Build history of the part. All positions in model axes, mm. A direction names the side the tool comes from. Coordinates: 2 decimals unless noted, no trailing zeros. Write each loop counter-clockwise with the first axis right and the second up, starting at its lowest first coordinate (ties: lowest second). Pieces come first, ordered by that corner, then holes.
from build123d import *

# Parameters (mm, degrees)
SKETCH1_W           = 19.05
SKETCH1_H           = 9.525
BOSS_EXTRUDE1_DEPTH = 3.175
SKETCH2_W           = 12.7
SKETCH2_H           = 9.525
BOSS_EXTRUDE2_DEPTH = 8.128
SKETCH3_W           = 6.35
SKETCH3_H           = 3.81
CUT_EXTRUDE1_DEPTH  = 18.584341301
FILLET1_START       = -4.7625
FILLET1_DEPTH       = 9.525
FILLET1_2_DEPTH     = 9.525
FILLET2_R           = 1.5875


with BuildPart() as part:
    # Sketch1 → Boss-Extrude1 (new body)
    with BuildSketch(Plane.XY):
        Rectangle(SKETCH1_W, SKETCH1_H)
    extrude(amount=BOSS_EXTRUDE1_DEPTH)

    # Sketch2 → Boss-Extrude2 (add)
    with BuildSketch(Plane.XY.offset(3.175)):
        Rectangle(SKETCH2_W, SKETCH2_H)
    extrude(amount=BOSS_EXTRUDE2_DEPTH)

    # Sketch3 → Cut-Extrude1 (cut, through all)
    with BuildSketch(Plane.XZ.offset(4.7625)):
        with Locations((0, 6.223)):
            Rectangle(SKETCH3_W, SKETCH3_H)
    extrude(amount=-CUT_EXTRUDE1_DEPTH, mode=Mode.SUBTRACT)

    # Fillet1: read off the stored shape, not the designer's step
    # Fillet1 outline → Fillet1 (cut)
    with BuildSketch(Plane(origin=(0, 0, 0), x_dir=(1, 0, 0), z_dir=(0, 1, 0)).offset(FILLET1_START)):
        with BuildLine():
            ThreePointArc((6.35, -8.128), (5.42006403, -10.37306403), (3.175, -11.303))
            Line((3.175, -11.303), (6.35, -11.303))
            Line((6.35, -11.303), (6.35, -8.128))
        make_face()
        with BuildLine():
            ThreePointArc((-3.175, -11.303), (-5.42006403, -10.37306403), (-6.35, -8.128))
            Line((-6.35, -8.128), (-6.35, -11.303))
            Line((-6.35, -11.303), (-3.175, -11.303))
        make_face()
    extrude(amount=FILLET1_DEPTH, mode=Mode.SUBTRACT)

    # Fillet1 2 outline → Fillet1 2 (add)
    with BuildSketch(Plane(origin=(0, 0, 0), x_dir=(1, 0, 0), z_dir=(0, 1, 0)).offset(FILLET1_START)):
        with BuildLine():
            Line((6.35, -3.175), (6.35, -6.35))
            ThreePointArc((6.35, -6.35), (7.27993597, -4.10493597), (9.525, -3.175))
            Line((9.525, -3.175), (6.35, -3.175))
        make_face()
        with BuildLine():
            ThreePointArc((-9.525, -3.175), (-7.27993597, -4.10493597), (-6.35, -6.35))
            Line((-6.35, -6.35), (-6.35, -3.175))
            Line((-6.35, -3.175), (-9.525, -3.175))
        make_face()
    extrude(amount=FILLET1_2_DEPTH)

    # Fillet2
    fillet2_edges = [part.edges().sort_by_distance(p)[0] for p in [
        (-9.525, 0, 3.175),
        (9.525, 0, 3.175),
    ]]
    fillet(fillet2_edges, radius=FILLET2_R)


solid = part.part
(1) 3-axis set-ups, long thin cutter, end or side, ignore diameter. For faces 1 (the flat face through (-3.175, 0, 6)), 2 (the cylindrical face through (5.445, -0.067, 10.348)), 3 (the flat face through (-6.35, 0, 7)): which of +Z, -Z, +X, -X, +Y, -Y reach the whole face in a straight line?
(2) Probe L1, parallel to Z at x = 1, y = -2; L2, parallel to X at y = 2.25, z = 7.5 (3 decimals); L3, parallel to Z at x = 5.5, y = 2.5. List the from-to ranges inside material, lowest first.
(3) Slice it at C-C, the plane z = 5. List the corners of the cut face in (x, y) (1 decimal), and give its area (3 significant figures).
(4) Two-plate mould, pull along X, no slides. Class faces 4 (the flat face through (0, -4.762, 4)), 5 (the flat face through (6.35, 0, 7)), 6 (the flat face through (0, 0, 4.318)): pulls with the +X half, pulls with the -X half, needs draft (parallel to the pull), parting line crosses it, or undercut.
(5) Flat gauge pins, fed straight in: P1, Ø1.9, axis at x = 1, y = 0, coming from the -Z side; P2, Ø3, axis at y = 1, z = 4.5, coming from the +X side; P3, Ø2, axis at y = 0, z = 7, coming from the -X side; P4, Ø1.9, axis at y = 0, z = 6.5, coming from the -X side. Where does each tip first touch, or does it go through?
(6) Slice it at D-D, the plane z = 3.75. List the corners of the cut face in (x, y), and give its area (3 significant figures).
(7) Slice it at A-A, the plane x = -1. List the corners of the cut face in (y, z).
Results:
1. face 1: +Y, -Y
1. face 2: +Z, +X, +Y, -Y
1. face 3: +Z, -X, +Y, -Y
2. L1: z = 0 to 4.32, 8.13 to 11.3
2. L2: x = -6.35 to -3.175, 3.175 to 6.35
2. L3: z = 0 to 10.29
3. outline: (-6.7, -4.8) - (-3.2, -4.8) - (-3.2, 4.8) - (-6.7, 4.8) - close; (3.2, -4.8) - (6.7, -4.8) - (6.7, 4.8) - (3.2, 4.8) - close
3. area: 66.2 mm2
4. face 4: needs draft
4. face 5: pulls with the +X half
4. face 6: undercut
5. P1: stops at z = 0
5. P2: stops at x = 9.04
5. P3: stops at x = -6.37
5. P4: stops at x = -6.45
6. outline: (-7.7, -4.76) - (7.7, -4.76) - (7.7, 4.76) - (-7.7, 4.76) - close
6. area: 147 mm2
7. outline: (-4.76, 0) - (4.76, 0) - (4.76, 4.32) - (-4.76, 4.32) - close; (-4.76, 8.13) - (4.76, 8.13) - (4.76, 11.3) - (-4.76, 11.3) - close
